Source: three-view drawing plus pictorial views. Frame: mm from the lowest corner of the part. A direction names the side the tool comes from. Round coordinates to 2 decimals unless told otherwise and drop trailing zeros. Loops run counter-clockwise (first coordinate to the right, second up) from the corner with the lowest first, then second, coordinate; pieces in that order, holes last. Notation, with made-up numbers: M 76,17 L 92,17 A14 ccw 92,28 Z; hole C 85,81 d8. An arc over 180 degrees is marked long. Return JSON: item names as keys, results as strings. Group by question number.
1) Access query for the marked faces 4, 5, 6, 7 and 8. Directions: +Z, -Z, +X, -X, +Y, -Y. A direction counts if a zero-diameter tool reaches every point of the face in a straight line with its end or side. Return the directions, or none.
2) Material intervals for line 1 (Y direction, x = 11.75, z = 2.5); line 2 (Y direction, x = 3, z = 3), sorted ascending. Write a range as from..to.
3) Section D-D (y = 8.5). Output: boundary loops of the cut face in (x, z), plus the area to 3 significant figures.
4) Mould query, pull axis Y, two halves, no side actions, for the marked faces 1, 2 and 3. Classes: +Y half, -Y half, draft (parallel to the pull), parting line (faces both ways), or undercut.
5) Contact query for flat-ended pins moving along their axis: P1, Ø1.5, axis at x = 2.5, z = 3.5, coming from the +Y side; P2, Ø1.5, axis at y = 3, z = 2.5, coming from the -X side; P3, Ø4, axis at y = 20.5, z = 2, coming from the -X side. Output: stop coordinate, or through.
6) Section B-B (x = 11.25). Output: boundary loops of the cut face in (y, z).
7) Section A-A (z = 3.25). Output: boundary loops of the cut face in (x, y).
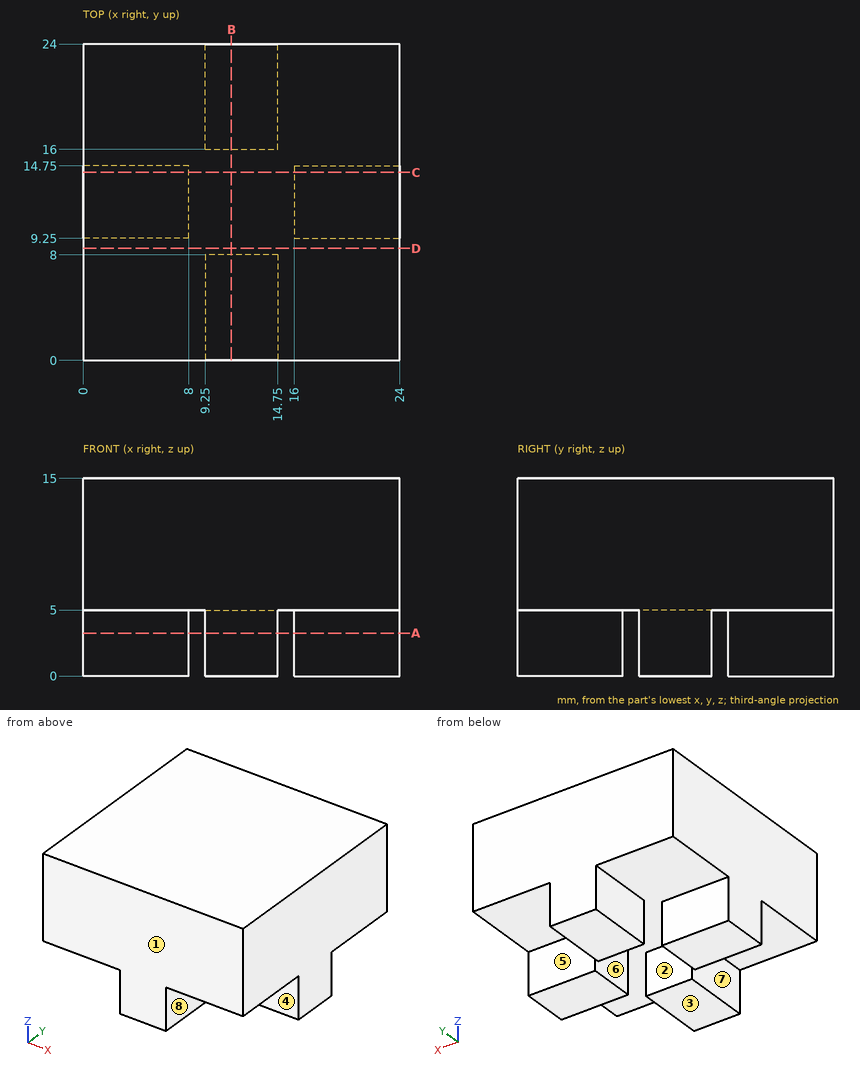
Returned:
{
 "1": {"face 4": "-Z, +X, -X, -Y", "face 5": "-Z, +X, -X, +Y", "face 6": "-Z, +Y, -Y", "face 7": "-Z, -X, +Y, -Y", "face 8": "-Z, +X, +Y, -Y"},
 "2": {"line 1": "y = 0..8, 16..24", "line 2": "y = 9.25..14.75"},
 "3": {"outline": "M 0,5 L 24,5 L 24,15 L 0,15 Z", "area": "240 mm^2"},
 "4": {"face 1": "-Y half", "face 2": "undercut", "face 3": "draft"},
 "5": {"P1": "stops at y = 14.75", "P2": "stops at x = 9.25", "P3": "stops at x = 9.25"},
 "6": {"outline": "M 0,0 L 8,0 L 8,5 L 16,5 L 16,0 L 24,0 L 24,15 L 0,15 Z"},
 "7": {"outline": "M 0,9.25 L 8,9.25 L 8,14.75 L 0,14.75 Z; M 9.25,0 L 14.75,0 L 14.75,8 L 9.25,8 Z; M 9.25,16 L 14.75,16 L 14.75,24 L 9.25,24 Z; M 16,9.25 L 24,9.25 L 24,14.75 L 16,14.75 Z"}
}
